Build history of the part. All positions in model axes, mm. Coordinates: 2 decimals unless noted, no trailing zeros. Loops run counter-clockwise (first coordinate to the right, second up) from the corner with the lowest first, then second, coordinate; pieces in that order, holes last. Notation, with made-up numbers: M -34.75,58 L 6.25,58 A9 cw 6.25,69 Z; hole C 89.5,-22 d11. An arc over 180 degrees is marked long. Write each question's results on one line, items separated by ' | '. Start each with the question number.
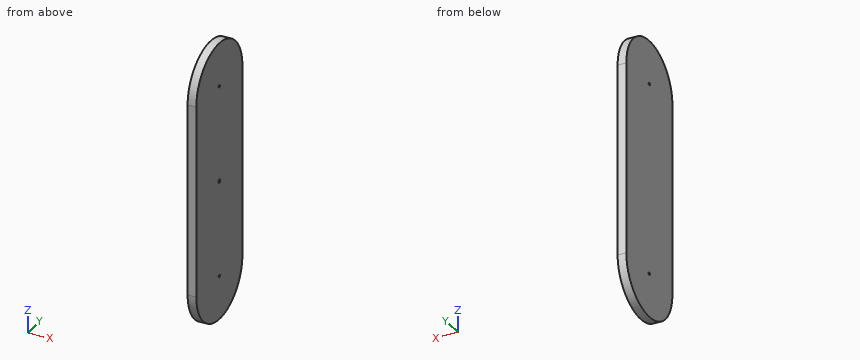
Autodesk Inventor part; units mm, degrees
ref_plane "YZ Plane" through (0, 0, 0) normal (1, 0, 0) x (0, 1, 0)
ref_plane "XZ Plane" through (0, 0, 0) normal (0, 1, 0) x (-1, 0, 0)
ref_plane "XY Plane" through (0, 0, 0) normal (0, 0, 1) x (1, 0, 0)
sketch "Sketch1" plane through (0, 0, 0) normal (1, 0, 0) x (0, 1, 0)
  arc A0 (-26.7534, -4.2636) -> (36.7466, -4.2636) centre (4.9966, -4.2636) ccw
  line L0 (36.7466, -4.2636) -> (36.7466, 65.5864)
  line L1 (-26.7534, -4.2636) -> (-26.7534, 65.5864)
  arc A1 (36.7466, 135.4364) -> (-26.7534, 135.4364) centre (4.9966, 135.4364) ccw
  line L2 (36.7466, 135.4364) -> (36.7466, 65.5864)
  line L3 (-26.7534, 135.4364) -> (-26.7534, 65.5864)
  circle A2 centre (4.9966, 135.4364) radius 0.9144
  circle A3 centre (4.9966, -4.2636) radius 0.9144
  dimension "d3" = 1.8288
  dimension "d4" = 1.8288
extrude "Extrusion1" add sketch "Sketch1" along normal blind 6.35
sketch "Sketch2" plane through (6.35, 0, 0) normal (1, 0, 0) x (0, 0, -1)
  point P0 (0, 0)
sketch "Sketch4" plane through (6.35, 0, 0) normal (1, 0, 0) x (0, 0, -1)
  circle A0 centre (-135.4364, 4.9966) radius 0.9144
  circle A1 centre (4.2636, 4.9966) radius 0.9144
  circle A2 centre (-65.5864, 4.9966) radius 1.27
  point P0 (0, 0)
  dimension "d14" = 2.54
extrude "Extrusion3" cut sketch "Sketch4" against normal blind 3 contours A2
properties part number "Second Arm"
1. Band-saw the part on A-A, the plane x = 1.25. List the corners of the cut face in (y, z).
2. Band-saw the part on B-B, the plane y = 18. List the corners of the cut face in (x, z).
3. Pin check, flat tips, straight feed: pin 1 (2 mm diameter, centred on x = 3.5, y = 8.5, fed in from -Z); pin 2 (2 mm diameter, centred on x = 4.5, y = 13.5, fed in from -Z). Stop position of each tip, or through.
4. Band-saw the part on C-C, the plane z = -19. List the corners of the cut face in (x, y), plus the area to 3 significant figures.
5. Wall check: line 1 along Z through (x, y) = (3.5, 5.5); line 2 along Z through (x, y) = (1, 3.5); line 3 along Z through (x, y) = (3, -20.5). Give the ranges that are in metal, low to high.
Checked values:
1) outline: M -26.75,-4.26 A31.75 ccw 36.75,-4.26 L 36.75,135.44 A31.75 ccw -26.75,135.44 Z; hole C 5,-4.26 d1.83; hole C 5,135.44 d1.83
2) outline: M 0,-33.23 L 6.35,-33.23 L 6.35,164.4 L 0,164.4 Z
3) pin 1: z = -35.91 | pin 2: z = -35.11
4) outline: M 0,-23.13 L 6.35,-23.13 L 6.35,33.12 L 0,33.12 Z | area: 357 mm²
5) line 1: -36.01 to -5.03, -3.5 to 64.42, 66.75 to 134.67, 136.2 to 167.18 | line 2: -35.98 to 167.15 | line 3: -23.18 to 154.36
